Model file for the job. Use its own axes, mm. Coordinates: 2 decimals unless noted, no trailing zeros. Answer in a Markdown table with one row per item. Add a question column.
Autodesk Inventor part; units mm, degrees
ref_plane "YZ Plane" through (0, 0, 0) normal (1, 0, 0) x (0, 1, 0)
ref_plane "XZ Plane" through (0, 0, 0) normal (0, 1, 0) x (-1, 0, 0)
ref_plane "XY Plane" through (0, 0, 0) normal (0, 0, 1) x (1, 0, 0)
sketch "Sketch1" plane through (0, 0, 0) normal (0, 0, 1) x (1, 0, 0)
  line L0 (0, 6) -> (211.4, 6)
  line L1 (211.4, 6) -> (211.4, -53)
  line L2 (211.4, -53) -> (0, -53)
  line L3 (0, -53) -> (0, 6)
  line L4 (214.4, 3) -> (214.4, 0)
  line L5 (37.85, -53) -> (0, -53)
  line L6 (0, 6) -> (211.4, 6)
  line L7 (211.4, 3) -> (211.4, 6)
  line L8 (0, -53) -> (0, -56)
  line L9 (0, -56) -> (211.4, -56)
  line L10 (211.4, -56) -> (211.4, -53)
  line L11 (211.4, -42.7143) -> (214.4, -42.7143)
  line L12 (214.4, -42.7143) -> (214.4, -7.2857)
  line L13 (214.4, -7.2857) -> (211.4, -7.2857)
  line L14 (-8.1633, -25) -> (265.4045, -25) construction
  line L15 (37.85, 3) -> (48.85, 3)
  line L16 (37.85, 3) -> (37.85, 0)
  line L17 (48.85, 0) -> (37.85, 0)
  line L18 (48.85, 3) -> (48.85, 0)
  line L19 (56.85, 3) -> (67.85, 3)
  line L20 (56.85, 3) -> (56.85, 0)
  line L21 (67.85, 0) -> (56.85, 0)
  line L22 (67.85, 3) -> (67.85, 0)
  line L23 (143.55, 3) -> (154.55, 3)
  line L24 (143.55, 3) -> (143.55, 0)
  line L25 (154.55, 0) -> (143.55, 0)
  line L26 (154.55, 3) -> (154.55, 0)
  line L27 (162.55, 3) -> (173.55, 3)
  line L28 (162.55, 3) -> (162.55, 0)
  line L29 (173.55, 0) -> (162.55, 0)
  line L30 (173.55, 3) -> (173.55, 0)
  line L31 (162.55, -50) -> (173.55, -50)
  line L32 (162.55, -50) -> (162.55, -53)
  line L33 (173.55, -53) -> (162.55, -53)
  line L34 (173.55, -50) -> (173.55, -53)
  line L35 (143.55, -50) -> (154.55, -50)
  line L36 (143.55, -50) -> (143.55, -53)
  line L37 (154.55, -53) -> (143.55, -53)
  line L38 (154.55, -50) -> (154.55, -53)
  line L39 (56.85, -50) -> (67.85, -50)
  line L40 (56.85, -50) -> (56.85, -53)
  line L41 (67.85, -53) -> (56.85, -53)
  line L42 (67.85, -50) -> (67.85, -53)
  line L43 (37.85, -50) -> (48.85, -50)
  line L44 (37.85, -50) -> (37.85, -53)
  line L45 (48.85, -53) -> (37.85, -53)
  line L46 (48.85, -50) -> (48.85, -53)
  line L47 (143.55, -53) -> (154.55, -53)
  line L48 (154.55, -53) -> (154.55, -50)
  line L49 (154.55, -50) -> (143.55, -50)
  line L50 (143.55, -50) -> (143.55, -53)
  line L51 (162.55, -53) -> (173.55, -53)
  line L52 (173.55, -53) -> (173.55, -50)
  line L53 (173.55, -50) -> (162.55, -50)
  line L54 (162.55, -50) -> (162.55, -53)
  line L55 (56.85, -53) -> (67.85, -53)
  line L56 (67.85, -53) -> (67.85, -50)
  line L57 (67.85, -50) -> (56.85, -50)
  line L58 (56.85, -50) -> (56.85, -53)
  line L59 (48.85, -53) -> (37.85, -53)
  line L60 (37.85, -53) -> (37.85, -50)
  line L61 (37.85, -50) -> (48.85, -50)
  line L62 (48.85, -50) -> (48.85, -53)
  line L63 (211.4, -56) -> (0, -56)
  line L64 (0, -56) -> (0, -53)
  line L65 (0, -53) -> (211.4, -53)
  line L66 (211.4, -53) -> (211.4, -56)
  line L67 (154.55, 0) -> (162.55, 3) construction
  line L68 (154.55, 3) -> (162.55, 0) construction
  line L69 (48.85, 3) -> (56.85, 0) construction
  line L70 (48.85, 0) -> (56.85, 3) construction
  line L71 (48.85, -50) -> (56.85, -53) construction
  line L72 (48.85, -53) -> (56.85, -50) construction
  line L73 (154.55, -53) -> (162.55, -50) construction
  line L74 (154.55, -50) -> (162.55, -53) construction
  circle A0 centre (158.55, 1.5) radius 1.4
  circle A1 centre (52.85, 1.5) radius 1.4
  circle A2 centre (52.85, -51.5) radius 1.4
  circle A3 centre (158.55, -51.5) radius 1.4
  point P0 (0, 0)
  dimension "d0" = 3
  dimension "d1" = 3
  dimension "d2" = 62
  dimension "d3" = 31
  dimension "d4" = 35.4286
  dimension "d7" = 2.8
  dimension "d8" = 2.8
  dimension "d9" = 2.8
  dimension "d10" = 2.8
extrude "Extrusion1" add sketch "Sketch1" along normal blind 3 contours L0 L1 L2 L34 L31 L32 L38 L35 L36 L42 L39 L40 L46 L43 L44 L3 | L2 L10 L9 L8 | L13 L12 L11 L1
equation "\"d3\" = 0.5 * d2"
equation "\"d4\" = 0.571429 * d2"
properties part number "slider-holder_side"
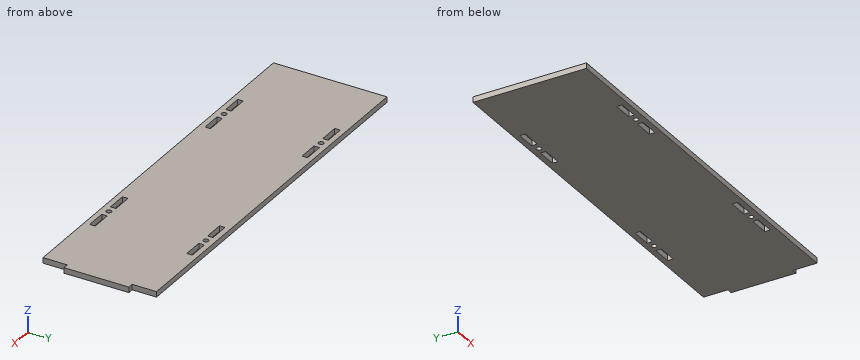
1) Flat gauge pins, fed straight in: pin 1 Ø3 at (x, y) = (169.5, -8) entering from -Z; pin 2 Ø1.5 at (y, z) = (1, 1) entering from +X. Where does each tip first touch, or does it go through?
2) Drill centre lines: probe 1 along Y at (x, z) = (154.5, 1.8); probe 2 along Y at (x, z) = (52.85, 1.3); probe 3 along X at (y, z) = (-5.5, 2.35). Where is each one in solid material? Low to high.
3) Slice it at A-A (z = 1.4). Count the separate pieces of the cut face and the enclosed holes in it, then the cut area to 3 significant figures.
Ans:
| question | item | result |
|---|---|---|
| 1 | pin 1 | stops at z = 0 |
| 1 | pin 2 | stops at x = 211.4 |
| 2 | probe 1 | y = -56 to -53, -50 to 0, 3 to 6 |
| 2 | probe 2 | y = -56 to -52.9, -50.1 to 0.1, 2.9 to 6 |
| 2 | probe 3 | x = 0 to 211.4 |
| 3 | separate pieces | 1 |
| 3 | enclosed holes | 12 |
| 3 | area | 12,900 mm2 |
